```python
from build123d import *

# Parameters (mm, degrees)
F0_W     = 215.9
F0_H     = 152.4
F1_DEPTH = 3.048
F2_W     = 25.4
F2_H     = 63.5
F2_R     = 34.925
F2_W_2   = 88.9
F2_H_2   = 19.05
F3_DEPTH = 25.4
F4_R     = 43.18
F5_R     = 5.08
F6_R     = 25.4


with BuildPart() as f1:
    # F0 (on Top) → F1 (new body)
    with BuildSketch(Plane.XY):
        Rectangle(F0_W, F0_H)
    extrude(amount=F1_DEPTH)

    # F2 (on Top) → F3 (cut)
    with BuildSketch(Plane.XY):
        with Locations((-76.2, 12.341094)):
            Rectangle(F2_W, F2_H)
        with Locations((-6.35, 19.05)):
            Circle(F2_R)
        with Locations((57.15, -32.164129)):
            Circle(F2_R)
        with Locations((-44.45, -41.275)):
            Rectangle(F2_W_2, F2_H_2)
    extrude(amount=F3_DEPTH, mode=Mode.SUBTRACT)

    # F4
    f4_edges = [f1.edges().sort_by_distance(p)[0] for p in [
        (-107.95, -76.2, 1.524),
        (107.95, -76.2, 1.524),
    ]]
    fillet(f4_edges, radius=F4_R)

    # F5
    f5_edges = [f1.edges().sort_by_distance(p)[0] for p in [
        (-88.9, 44.091094, 1.524),
        (-63.5, 44.091094, 1.524),
        (-88.9, -19.408906, 1.524),
        (-63.5, -19.408906, 1.524),
        (0, -50.8, 1.524),
        (0, -31.75, 1.524),
        (-88.9, -50.8, 1.524),
        (-88.9, -31.75, 1.524),
    ]]
    fillet(f5_edges, radius=F5_R)

    # F6
    f6_edges = [f1.edges().sort_by_distance(p)[0] for p in [
        (-107.95, 76.2, 1.524),
        (107.95, 76.2, 1.524),
    ]]
    fillet(f6_edges, radius=F6_R)


solid = f1.part
```
Can you work these out from the model? Positions are in its coordinate system, mm. A direction names the side the tool comes from. Coordinates: 2 decimals unless noted, no trailing zeros. Write each loop counter-clockwise with the first axis right and the second up, starting at its lowest first coordinate (ties: lowest second). Pieces come first, ordered by that corner, then holes. Notation, with made-up numbers: M -37,74.5 L 12,74.5 A24 ccw 12,86.5 Z; hole C 87,77 d7. An arc over 180 degrees is marked long. Answer as CSV lines item,"result".
Item 1: Imagine slicing it at D-D on y = -58. List the corners of the cut face in (x, z) for me.
Geometry results:
outline,"M -99.99,0 L 33.65,0 L 33.65,3.05 L -99.99,3.05 Z; M 80.65,0 L 99.99,0 L 99.99,3.05 L 80.65,3.05 Z"
Item 2: We'd pull the mould along Y, two halves only. Please class faces 1 (the cylindrical face through (-1.449, -33.278, 1.545)), 2 (the cylindrical face through (-100.71, 68.56, 1.55)), 3 (the cylindrical face through (-87.37, -17.96, 1.55)), 4 (the cylindrical face through (-95.637, -63.215, 1.545)): +Y half, -Y half, draft (parallel to the pull), parting line (faces both ways), or undercut.
Geometry results:
face 1,"undercut"
face 2,"+Y half"
face 3,"undercut"
face 4,"-Y half"
Item 3: I'm going to push a flat-ended pin straight in: P1, Ø1.5, axis at y = -42.5, z = 1, coming from the +X side. Where does the tip first touch, or does it pass through?
Geometry results:
P1,"stops at x = 107.06"
Item 4: On a 3-axis mill with a long thin cutter (end or side, diameter ignored), from which of +Z, -Z, +X, -X, +Y, -Y can I reach the whole of each face in a straight line? I mean faces 5 (the cylindrical face through (-87.372, -49.351, 1.545)), 6 (the flat face through (-2, -16, 0)). Say none if no direction works.
Geometry results:
face 5,"+Z, -Z"
face 6,"-Z, +X, -X, +Y, -Y"
Item 5: Imagine slicing it at C-C on x = -22. List the corners of the cut face in (y, z) for me.
Geometry results:
outline,"M -76.2,0 L -50.8,0 L -50.8,3.05 L -76.2,3.05 Z; M -31.75,0 L -12.17,0 L -12.17,3.05 L -31.75,3.05 Z; M 50.27,0 L 76.2,0 L 76.2,3.05 L 50.27,3.05 Z"
Item 6: Imagine slicing it at A-A on x = 57.15. List the corners of the cut face in (y, z) for me.
Geometry results:
outline,"M -76.2,0 L -67.09,0 L -67.09,3.05 L -76.2,3.05 Z; M 2.76,0 L 76.2,0 L 76.2,3.05 L 2.76,3.05 Z"
Item 7: Please list where these lines run through material, in increasing order: line 1 along X through (y, z) = (19.05, 0.7) (3 decimals); line 2 along Y through (x, z) = (-6.35, 1.5) (3 decimals); line 3 along X through (y, z) = (23.5, 1.25).
Geometry results:
line 1,"x = -107.95 to -88.9, -63.5 to -41.275, 28.575 to 107.95"
line 2,"y = -76.2 to -50.8, -31.75 to -15.875, 53.975 to 76.2"
line 3,"x = -107.95 to -88.9, -63.5 to -40.99, 28.29 to 107.95"
Item 8: Imagine slicing it at B-B on y = 19.05. List the corners of the cut face in (x, z) for me (3 decimals).
Geometry results:
outline,"M -107.95,0 L -88.9,0 L -88.9,3.048 L -107.95,3.048 Z; M -63.5,0 L -41.275,0 L -41.275,3.048 L -63.5,3.048 Z; M 28.575,0 L 107.95,0 L 107.95,3.048 L 28.575,3.048 Z"
